Geometry: final body of the model. Coordinates: model frame, mm. A direction names the side the tool comes from. Give positions to 0.01 mm unless a question says otherwise; leave off trailing zeros. Loops run counter-clockwise (first coordinate to the right, second up) from the corner with the lowest first, then second, coordinate; pieces in that order, holes last.
from build123d import *

# Parameters (mm, degrees)
EXTRUDE_1_DEPTH     = 1
SKETCH_2_R          = 1.6
CUT_EXTRUDE_1_DEPTH = 4
FILLET_3_R          = 2
FILLET_4_R          = 2
FILLET_5_R          = 2
FILLET_6_R          = 2
FILLET_7_R          = 2
FILLET_8_R          = 2
FILLET_9_R          = 2
FILLET_10_R         = 2


with BuildPart() as part:
    # 草图1 → 凸台-拉伸1 (new body)
    with BuildSketch(Plane.XY):
        with BuildLine():
            Line((-34.555089852, 10.529608301), (-34.555089852, 26))
            Line((-34.555089852, 26), (-44.5, 26))
            Line((-44.5, 26), (-44.5, -26))
            Line((-44.5, -26), (-34.555089852, -26))
            Line((-34.555089852, -26), (-34.555089852, -10.529608301))
            add(Edge.make_bspline(
                [(-34.555089852, -10.529608301), (-34.215666053, -8.393494982), (-32.082061244, -5.04423915), (-29.471557065, -5.067226444)],
                knots=[0, 0, 0, 0, 1, 1, 1, 1], degree=3))
            Line((-29.471557065, -5.067226444), (29.471557065, -5.067226444))
            add(Edge.make_bspline(
                [(34.555089852, -10.529608301), (34.215666053, -8.393494982), (32.082061244, -5.04423915), (29.471557065, -5.067226444)],
                knots=[0, 0, 0, 0, 1, 1, 1, 1], degree=3))
            Line((34.555089852, -10.529608301), (34.555089852, -26))
            Line((34.555089852, -26), (44.5, -26))
            Line((44.5, -26), (44.5, 26))
            Line((44.5, 26), (34.555089852, 26))
            Line((34.555089852, 26), (34.555089852, 10.529608301))
            add(Edge.make_bspline(
                [(34.555089852, 10.529608301), (34.215666053, 8.393494982), (32.082061244, 5.04423915), (29.471557065, 5.067226444)],
                knots=[0, 0, 0, 0, 1, 1, 1, 1], degree=3))
            Line((29.471557065, 5.067226444), (-29.471557065, 5.067226444))
            add(Edge.make_bspline(
                [(-34.555089852, 10.529608301), (-34.215666053, 8.393494982), (-32.082061244, 5.04423915), (-29.471557065, 5.067226444)],
                knots=[0, 0, 0, 0, 1, 1, 1, 1], degree=3))
        make_face()
    extrude(amount=-EXTRUDE_1_DEPTH)

    # 草图2 → 切除-拉伸1 (cut)
    with BuildSketch(Plane.XY):
        with Locations((-39.5, 21)):
            Circle(SKETCH_2_R)
        with Locations((39.5, 21)):
            Circle(SKETCH_2_R)
        with Locations((-39.5, -21)):
            Circle(SKETCH_2_R)
        with Locations((39.5, -21)):
            Circle(SKETCH_2_R)
    extrude(amount=-CUT_EXTRUDE_1_DEPTH, mode=Mode.SUBTRACT)

    # 圆角3
    fillet_3_edges = [part.edges().sort_by_distance(p)[0] for p in [
        (-44.5, 26, -0.5),
    ]]
    fillet(fillet_3_edges, radius=FILLET_3_R)

    # 圆角4
    fillet_4_edges = [part.edges().sort_by_distance(p)[0] for p in [
        (-34.555089852, 26, -0.5),
    ]]
    fillet(fillet_4_edges, radius=FILLET_4_R)

    # 圆角5
    fillet_5_edges = [part.edges().sort_by_distance(p)[0] for p in [
        (-44.5, -26, -0.5),
    ]]
    fillet(fillet_5_edges, radius=FILLET_5_R)

    # 圆角6
    fillet_6_edges = [part.edges().sort_by_distance(p)[0] for p in [
        (-34.555089852, -26, -0.5),
    ]]
    fillet(fillet_6_edges, radius=FILLET_6_R)

    # 圆角7
    fillet_7_edges = [part.edges().sort_by_distance(p)[0] for p in [
        (34.555089852, -26, -0.5),
    ]]
    fillet(fillet_7_edges, radius=FILLET_7_R)

    # 圆角8
    fillet_8_edges = [part.edges().sort_by_distance(p)[0] for p in [
        (44.5, -26, -0.5),
    ]]
    fillet(fillet_8_edges, radius=FILLET_8_R)

    # 圆角9
    fillet_9_edges = [part.edges().sort_by_distance(p)[0] for p in [
        (34.555089852, 26, -0.5),
    ]]
    fillet(fillet_9_edges, radius=FILLET_9_R)

    # 圆角10
    fillet_10_edges = [part.edges().sort_by_distance(p)[0] for p in [
        (44.5, 26, -0.5),
    ]]
    fillet(fillet_10_edges, radius=FILLET_10_R)


solid = part.part
Item 1: Draft query along Y for faces 4 (the face through (39.292, -19.414, -0.493)), 5 (the face through (35.125, -25.399, -0.507)), 6 (the face through (0, 2, -1)). Return one class per face: +Y half, -Y half, draft (parallel to the pull), parting line (faces both ways), or undercut.
Values follow:
face 4: undercut
face 5: -Y half
face 6: draft
Item 2: Section query A-A on y = -21. Return loops of the section in (x, z), plus the area to 3 significant figures.
Values follow:
outline: (-44.5, -1) - (-41.1, -1) - (-41.1, 0) - (-44.5, 0) - close; (-37.9, -1) - (-34.56, -1) - (-34.56, 0) - (-37.9, 0) - close; (34.56, -1) - (37.9, -1) - (37.9, 0) - (34.56, 0) - close; (41.1, -1) - (44.5, -1) - (44.5, 0) - (41.1, 0) - close
area: 13.5 mm2
Item 3: Section query C-C on y = 12.5. Return loops of the section in (x, z).
Values follow:
outline: (-44.5, -1) - (-34.56, -1) - (-34.56, 0) - (-44.5, 0) - close; (34.56, -1) - (44.5, -1) - (44.5, 0) - (34.56, 0) - close
Item 4: Section query B-B on x = -39.5. Return loops of the section in (y, z), plus the area to 3 significant figures.
Values follow:
outline: (-26, -1) - (-22.6, -1) - (-22.6, 0) - (-26, 0) - close; (-19.4, -1) - (19.4, -1) - (19.4, 0) - (-19.4, 0) - close; (22.6, -1) - (26, -1) - (26, 0) - (22.6, 0) - close
area: 45.6 mm2
Item 5: Section query D-D on z = -0.2. Give the number of separate pieces and of enclosed holes in the cut face, plus the area to 3 significant figures.
Values follow:
separate pieces: 1
enclosed holes: 4
area: 1,730 mm2
Item 6: Pin query (flat end, axial travel): pin 1 (12 mm diameter, centred on x = -19, y = 11.5, fed in from +Z); pin 2 (0.5 mm diameter, centred on x = -6.5, z = -0.5, fed in from +Y). Return the tip coordinate at first contact, or that it passes through.
Values follow:
pin 1: passes through
pin 2: stops at y = 5.07
Item 7: Ray query, probe 1 along Y at (x, z) = (39.5, -0.4); probe 2 along X at (y, z) = (-11, -0.25); probe 3 along X at (y, z) = (-20, -0.1). Return the intervals inside material, ascending.
Values follow:
probe 1: y = -26 to -22.6, -19.4 to 19.4, 22.6 to 26
probe 2: x = -44.5 to -34.56, 34.56 to 44.5
probe 3: x = -44.5 to -40.75, -38.25 to -34.56, 34.56 to 38.25, 40.75 to 44.5
Item 8: Set-up query: faces 1 (the face through (-35.157, -25.43, -0.507)), 2 (the face through (35.157, 25.43, -0.507)), 3 (the face through (0, 2, 0)). Return all of +Z, -Z, +X, -X, +Y, -Y with unobstructed straight access to the full face (end or side cutting, diameter ignored); none if empty.
Values follow:
face 1: +Z, -Z, -Y
face 2: +Z, -Z, +Y
face 3: +Z, +X, -X, +Y, -Y
